```python
from build123d import *

# Parameters (mm, degrees)
SKETCH1_W           = 135
SKETCH1_H           = 73
BOSS_EXTRUDE1_DEPTH = 2
SKETCH2_W           = 2
SKETCH2_H           = 73
BOSS_EXTRUDE2_DEPTH = 50
SKETCH4_W           = 8
SKETCH4_H           = 8
SKETCH4_R           = 2.5
SKETCH4_W_2         = 10
SKETCH4_H_2         = 10
SKETCH4_W_3         = 5
SKETCH4_H_3         = 5
BOSS_EXTRUDE4_DEPTH = 25
SKETCH5_R           = 2.5
CUT_EXTRUDE1_DEPTH  = 2
SKETCH6_R           = 3.75
CUT_EXTRUDE2_DEPTH  = 2
SKETCH7_W           = 5
SKETCH7_H           = 10
CUT_EXTRUDE3_DEPTH  = 2
SKETCH8_W           = 2
SKETCH8_H           = 9
BOSS_EXTRUDE5_DEPTH = 8
SKETCH9_R           = 2.5
CUT_EXTRUDE4_DEPTH  = 8
SKETCH10_R          = 2.5
CUT_EXTRUDE5_DEPTH  = 2


with BuildPart() as part:
    # Sketch1 → Boss-Extrude1 (new body)
    with BuildSketch(Plane(origin=(0, 0, 0), x_dir=(1, 0, 0), z_dir=(0, 1, 0))):
        Rectangle(SKETCH1_W, SKETCH1_H)
    extrude(amount=BOSS_EXTRUDE1_DEPTH)

    # Sketch2 → Boss-Extrude2 (add)
    with BuildSketch(Plane(origin=(0, 2, 0), x_dir=(1, 0, 0), z_dir=(0, 1, 0))):
        with Locations((-66.5, 0)):
            Rectangle(SKETCH2_W, SKETCH2_H)
    extrude(amount=BOSS_EXTRUDE2_DEPTH)

    # Sketch4 → Boss-Extrude4 (add)
    with BuildSketch(Plane(origin=(0, 2, 0), x_dir=(1, 0, 0), z_dir=(0, 1, 0))):
        with Locations((27.5, -27.5)):
            Rectangle(SKETCH4_W, SKETCH4_H)
        with Locations((27, -27)):
            Circle(SKETCH4_R, mode=Mode.SUBTRACT)
        with Locations((-59.5, -26.5)):
            Rectangle(SKETCH4_W_2, SKETCH4_H_2)
        with Locations((-58, -25)):
            Circle(SKETCH4_R, mode=Mode.SUBTRACT)
        with Locations((-59.5, 26.5)):
            Rectangle(SKETCH4_W_2, SKETCH4_H_2)
        with Locations((-58, 26)):
            Circle(SKETCH4_R, mode=Mode.SUBTRACT)
        with Locations((29, 29)):
            Rectangle(SKETCH4_W_3, SKETCH4_H_3)
    extrude(amount=BOSS_EXTRUDE4_DEPTH)

    # Sketch5 → Cut-Extrude1 (cut)
    with BuildSketch(Plane(origin=(0, 2, 0), x_dir=(1, 0, 0), z_dir=(0, 1, 0))):
        with Locations((9.5, -13.5)):
            Circle(SKETCH5_R)
    extrude(amount=-CUT_EXTRUDE1_DEPTH, mode=Mode.SUBTRACT)

    # Sketch6 → Cut-Extrude2 (cut)
    with BuildSketch(Plane(origin=(-65.5, 0, 0), x_dir=(0, 0, -1), z_dir=(1, 0, 0))):
        with Locations((-16.5, 40)):
            Circle(SKETCH6_R)
        with Locations((-5.5, 40)):
            Circle(SKETCH6_R)
        with Locations((5.5, 40)):
            Circle(SKETCH6_R)
        with Locations((16.5, 40)):
            Circle(SKETCH6_R)
    extrude(amount=-CUT_EXTRUDE2_DEPTH, mode=Mode.SUBTRACT)

    # Sketch7 → Cut-Extrude3 (cut)
    with BuildSketch(Plane(origin=(-65.5, 0, 0), x_dir=(0, 0, -1), z_dir=(1, 0, 0))):
        with Locations((-27, 39)):
            Rectangle(SKETCH7_W, SKETCH7_H)
    extrude(amount=-CUT_EXTRUDE3_DEPTH, mode=Mode.SUBTRACT)

    # Sketch8 → Boss-Extrude5 (add)
    with BuildSketch(Plane(origin=(0, 2, 0), x_dir=(1, 0, 0), z_dir=(0, 1, 0))):
        with Locations((66.5, 0)):
            Rectangle(SKETCH8_W, SKETCH8_H)
    extrude(amount=BOSS_EXTRUDE5_DEPTH)

    # Sketch9 → Cut-Extrude4 (cut)
    with BuildSketch(Plane(origin=(67.5, 0, 0), x_dir=(0, 0, -1), z_dir=(1, 0, 0))):
        with Locations((0, 6)):
            Circle(SKETCH9_R)
    extrude(amount=-CUT_EXTRUDE4_DEPTH, mode=Mode.SUBTRACT)

    # Sketch10 → Cut-Extrude5 (cut)
    with BuildSketch(Plane.ZY.offset(67.5)):
        with Locations((0, 47)):
            Circle(SKETCH10_R)
    extrude(amount=-CUT_EXTRUDE5_DEPTH, mode=Mode.SUBTRACT)


solid = part.part
```
Input: part model. Units: mm. Frame: model coordinates. A direction names the side the tool comes from. Coordinates: 2 decimals unless noted, no trailing zeros. Order: outer loops, then holes, each group sorted by start corner. A loop starts at its lowest first (then second) coordinate and runs counter-clockwise, first axis right, second up. Notation, with made-up numbers: (4, 16) - (53, 16) arc R29 ccw to (53, 41) - close; hole circle Ø5 at (64, -1). An arc over 180 degrees is marked (long way). Put each result on its own line as item: value.
1. Draft query along X for faces 1 (the face through (-67.5, 26, 1)), 2 (the face through (27, 2, 27)), 3 (the face through (-61, 27, 26)). Return one class per face: pulls with the +X half, pulls with the -X half, needs draft (parallel to the pull), parting line crosses it, or undercut.
Report:
face 1: pulls with the -X half
face 2: undercut
face 3: needs draft
2. Cut plane D-D on y = 29. Return the cut outline in (x, z).
Report:
outline: (-67.5, -36.5) - (-65.5, -36.5) - (-65.5, 36.5) - (-67.5, 36.5) - close
3. Line query: line 1 along Z through (x, y) = (-58, 11); line 2 along Y through (x, z) = (-66.25, 5.5); line 3 along X through (y, z) = (0.7, 13.5). Output: solid intervals per line, ascending.
Report:
line 1: z = -31.5 to -28.5, -23.5 to -21.5, 21.5 to 22.5, 27.5 to 31.5
line 2: y = 0 to 36.25, 43.75 to 52
line 3: x = -67.5 to 7, 12 to 67.5
4. Cut plane C-C on x = -32. Return the cut outline in (y, z), then the cut area to 3 significant figures.
Report:
outline: (0, -36.5) - (2, -36.5) - (2, 36.5) - (0, 36.5) - close
area: 146 mm2
5. Contact query for flat-ended pins moving along their axis: pin 1 Ø3 at (x, z) = (27, 27) entering from -Y; pin 2 Ø2 at (x, y) = (66, 7.5) entering from +Z; pin 3 Ø3 at (y, z) = (16, -24.5) entering from +X; pin 4 Ø2 at (x, z) = (-44.5, -16.5) entering from +Y. Output: stop coordinate, or through.
Report:
pin 1: stops at y = 0
pin 2: stops at z = 4.5
pin 3: stops at x = -54.5
pin 4: stops at y = 2
6. Reachability of faces 4 (the face through (27, 14, 23.5)), 5 (the face through (29, 14, -31.5)), 6 (the face through (-65.5, 27, 1)), 7 (the face through (-56.66, 14.32, 22.89)) from +Z, -Z, +X, -X, +Y, -Y: full face, straight path, thin tool, end or side. Return the list, or none.
Report:
face 4: +X, +Y
face 5: -Z, +X, +Y
face 6: +Z, -Z, +Y
face 7: +Y
7. Cut plane A-A on z = 0. Return the cut outline in (x, y), then the cut area to 3 significant figures.
Report:
outline: (-67.5, 0) - (67.5, 0) - (67.5, 3.5) - (65.5, 3.5) - (65.5, 2) - (-65.5, 2) - (-65.5, 44.5) - (-67.5, 44.5) - close; (-67.5, 49.5) - (-65.5, 49.5) - (-65.5, 52) - (-67.5, 52) - close; (65.5, 8.5) - (67.5, 8.5) - (67.5, 10) - (65.5, 10) - close
area: 366 mm2
8. Cut plane B-B on x = 9. Return the cut outline in (y, z), then the cut area to 3 significant figures.
Report:
outline: (0, -36.5) - (2, -36.5) - (2, 11.05) - (0, 11.05) - close; (0, 15.95) - (2, 15.95) - (2, 36.5) - (0, 36.5) - close
area: 136 mm2
